CAD build for the part. Positions are in the model's coordinates, mm. A direction names the side the tool comes from. Give positions to 0.01 mm unless a question says otherwise; leave off trailing zeros. Order: outer loops, then holes, each group sorted by start corner. A loop starts at its lowest first (then second) coordinate and runs counter-clockwise, first axis right, second up. Notation, with made-up numbers: (65, -32.75) -> (83, -32.75) arc R15 cw to (83, -27.75) -> close; hole circle Ø11 at (80, 29). An arc over 180 degrees is marked (long way). Use one line per item in the form item = value. Start each with the question number.
1) Cut at D-D, the plane z = 12.25. Give the cut face in (x, y), and give its area (3 significant figures).
2) Mould opens along X. For faces 4 (the face through (-4, 5, 10)), 5 (the face through (15.89, 6.28, 2.32)), 6 (the face through (25, 5, 2)), 7 (the face through (5.3, 4.9, -8.19)) say: pulls with the +X half, pulls with the -X half, needs draft (parallel to the pull), parting line crosses it, or undercut.
3) Tool access for faces 1 (the face through (-8.42, -1, -9)), 2 (the face through (-5, -1, 0)), 3 (the face through (-8.42, 11, -9)): list every direction of +Z, -Z, +X, -X, +Y, -Y with a clear straight run to the whole face (end or side of a thin tool).
4) Cut at A-A, the plane y = 3. State how many separate pieces and enclosed holes the cut face has, and give its area (3 significant figures).
5) Probe line 1 (X direction, y = 5, z = 0.5); line 2 (X direction, y = 7.25, z = -7); line 3 (Y direction, x = -21, z = -4). List the from-to ranges inside material, lowest first.
6) Cut at C-C, the plane x = -5.5. Give the cut face in (y, z).
7) Cut at B-B, the plane z = -7. Give the cut face in (x, y), and give its area (3 significant figures).
8) Drop flat-ended pins along their axis: P1, Ø2, axis at x = 17.5, y = 2.5, coming from the -Z side; P2, Ø1.6, axis at y = 10.5, z = 8, coming from the -X side; P3, Ø2.5, axis at x = 6.21, z = -7, coming from the -Y side; P4, Ø12, axis at x = -17, z = 9, coming from the -Y side. Give the stop position or say it passes through.
from build123d import *

# Parameters (mm, degrees)
SKETCH1_W           = 50
SKETCH1_H           = 20
BOSS_EXTRUDE1_DEPTH = 10
FILLET1_R           = 10
SKETCH2_R           = 2
CUT_EXTRUDE1_DEPTH  = 10
SKETCH4_R           = 3.35
CUT_EXTRUDE2_DEPTH  = 40
BOSS_EXTRUDE3_DEPTH = 2
SKETCH7_R           = 1.5
CUT_EXTRUDE3_DEPTH  = 20
FILLET3_R           = 2
FILLET4_R           = 1
SKETCH8_R           = 3.35
BOSS_EXTRUDE4_DEPTH = 5
CHAMFER1_SIZE       = 5


with BuildPart() as part:
    # Sketch1 → Boss-Extrude1 (new body)
    with BuildSketch(Plane(origin=(0, 0, 0), x_dir=(1, 0, 0), z_dir=(0, 1, 0))):
        Rectangle(SKETCH1_W, SKETCH1_H)
    extrude(amount=BOSS_EXTRUDE1_DEPTH)

    # Fillet1
    fillet1_edges = [part.edges().sort_by_distance(p)[0] for p in [
        (-25, 5, 10),
        (-25, 5, -10),
    ]]
    fillet(fillet1_edges, radius=FILLET1_R - 0.0001)  # a hair under: the kernel refuses the full size

    # Sketch2 → Cut-Extrude1 (cut)
    with BuildSketch(Plane(origin=(0, 10, 0), x_dir=(1, 0, 0), z_dir=(0, 1, 0))):
        with Locations(Location((-15, 0, 0), (0, 0, 270))):
            Circle(SKETCH2_R)
    extrude(amount=-CUT_EXTRUDE1_DEPTH, mode=Mode.SUBTRACT)

    # Sketch4 → Cut-Extrude2 (cut)
    with BuildSketch(Plane(origin=(0, 0, -10), x_dir=(-1, 0, 0), z_dir=(0, 0, -1))):
        with Locations((-18.984247751, 5)):
            Circle(SKETCH4_R)
    extrude(amount=-CUT_EXTRUDE2_DEPTH, mode=Mode.SUBTRACT)

    # Sketch6 → Boss-Extrude3 (add)
    with BuildSketch(Plane(origin=(0, 10, 0), x_dir=(1, 0, 0), z_dir=(0, 1, 0))):
        with BuildLine():
            Line((-8.420233762, 10), (-8.420233762, 7.53038354))
            ThreePointArc((-8.420233762, 7.53038354), (-5, 0), (-8.420233762, -7.53038354))
            Line((-8.420233762, -7.53038354), (-8.420233762, -10))
            Line((-8.420233762, -10), (25, -10))
            Line((25, -10), (25, 10))
            Line((25, 10), (-8.420233762, 10))
        make_face()
    boss_extrude3 = extrude(amount=BOSS_EXTRUDE3_DEPTH)

    # Sketch7 → Cut-Extrude3 (cut)
    with BuildSketch(Plane(origin=(0, 12, 0), x_dir=(1, 0, 0), z_dir=(0, 1, 0))):
        with Locations(Location((6.210160934, 7, 0), (0, 0, 270))):
            Circle(SKETCH7_R)
    cut_extrude3 = extrude(amount=-CUT_EXTRUDE3_DEPTH, mode=Mode.SUBTRACT)

    # Mirror3: Boss-Extrude3, Cut-Extrude3 across plane
    add(boss_extrude3.mirror(Plane(origin=(0, 5, 0), x_dir=(0, 0, 1), z_dir=(0, -1, 0))))
    add(cut_extrude3.mirror(Plane(origin=(0, 5, 0), x_dir=(0, 0, 1), z_dir=(0, -1, 0))), mode=Mode.SUBTRACT)

    # Fillet3
    fillet3_edges = [part.edges().sort_by_distance(p)[0] for p in [
        (25, 12, 0),
        (25, -2, 0),
    ]]
    fillet(fillet3_edges, radius=FILLET3_R)

    # Fillet4
    fillet4_edges = [part.edges().sort_by_distance(p)[0] for p in [
        (-15, 0, -2),
        (-15, 10, -2),
    ]]
    fillet(fillet4_edges, radius=FILLET4_R)

    # Sketch8 → Boss-Extrude4 (add)
    with BuildSketch(Plane.XY.offset(10)):
        with BuildLine():
            Line((12.964247751, 12), (12.964247751, -2))
            Line((12.964247751, -2), (23, -2))
            ThreePointArc((23, -2), (24.414213562, -1.414213562), (25, 0))
            Line((25, 0), (25, 10))
            ThreePointArc((25, 10), (24.414213562, 11.414213562), (23, 12))
            Line((23, 12), (12.964247751, 12))
        make_face()
        with Locations(Location((18.984247751, 5, 0), (0, 0, 180))):
            Circle(SKETCH8_R, mode=Mode.SUBTRACT)
    extrude(amount=BOSS_EXTRUDE4_DEPTH)

    # Chamfer1
    chamfer1_edges = [part.edges().sort_by_distance(p)[0] for p in [
        (12.964247751, 5, 10),
    ]]
    chamfer(chamfer1_edges, length=CHAMFER1_SIZE - 0.0001)  # a hair under: the kernel refuses the full size


solid = part.part
Result:
q1.outline = (10.21, -2) -> (23, -2) arc R2 ccw to (25, 0) -> (25, 10) arc R2 ccw to (23, 12) -> (10.21, 12) -> close; hole circle Ø6.7 at (18.98, 5)
q1.area = 170 mm²
q2.face_4 = needs draft
q2.face_5 = undercut
q2.face_6 = pulls with the +X half
q2.face_7 = undercut
q3.face_1 = +Z, -Z, -X, -Y
q3.face_2 = -X, -Y
q3.face_3 = +Z, -Z, -X, +Y
q4.separate_pieces = 2
q4.enclosed_holes = 2
q4.area = 876 mm²
q5.line_1 = -24.99 to -16.94, -13.06 to 15.63, 22.33 to 25
q5.line_2 = -22.14 to 4.71, 7.71 to 16.5, 21.47 to 25
q5.line_3 = 0 to 10
q6.outline = (-2, -10) -> (12, -10) -> (12, -3.12) -> (10, -3.12) -> (10, 3.12) -> (12, 3.12) -> (12, 10) -> (-2, 10) -> (-2, 3.12) -> (0, 3.12) -> (0, -3.12) -> (-2, -3.12) -> close
q7.outline = (-22.14, 0) -> (-7.86, 0) -> (-7.86, -2) -> (4.71, -2) -> (4.71, 12) -> (-7.86, 12) -> (-7.86, 10) -> (-22.14, 10) -> close; (7.71, -2) -> (23, -2) arc R2 ccw to (25, 0) -> (25, 10) arc R2 ccw to (23, 12) -> (7.71, 12) -> close; hole circle Ø6.7 at (18.98, 5)
q7.area = 524 mm²
q8.P1 = -10
q8.P2 = -21.75
q8.P3 = through
q8.P4 = 0
